```python
from build123d import *

# Parameters (mm, degrees)
BOSS_EXTRUDE1_DEPTH                            = 3
CSK_FOR_M4_FLAT_HEAD_MACHINE_SCREW7_AT_2_COUNT = 2
CSK_FOR_M4_FLAT_HEAD_MACHINE_SCREW7_AT_2_PITCH = 14.1
CSK_FOR_M4_FLAT_HEAD_MACHINE_SCREW7_AT_3_COUNT = 2
CSK_FOR_M4_FLAT_HEAD_MACHINE_SCREW7_AT_3_PITCH = 14.1


with BuildPart() as part:
    # Sketch2 → Boss-Extrude1 (new body)
    with BuildSketch(Plane(origin=(0, 0, 0), x_dir=(1, 0, 0), z_dir=(0, 1, 0))):
        with BuildLine():
            Line((14, -6), (-14, -6))
            ThreePointArc((-14, -6), (-20, 0), (-14, 6))
            Line((-14, 6), (14, 6))
            ThreePointArc((14, 6), (20, 0), (14, -6))
        make_face()
    extrude(amount=-BOSS_EXTRUDE1_DEPTH)

    # Sketch22 → CSK for M4 Flat Head Machine Screw7 (revolve, cut)
    with BuildSketch(Plane(origin=(0, 0, 0), x_dir=(0, 0, 1), z_dir=(1, 0, 0))):
        Polygon((0, 0), (0, 3), (2.25, 3), (2.25, 2.45), (4.7, 0), align=None)
    csk_for_m4_flat_head_machine_screw7 = revolve(axis=Axis((0, 6.35, 0), (0, -1, 0)), mode=Mode.SUBTRACT)

    # CSK for M4 Flat Head Machine Screw7 at 2: CSK for M4 Flat Head Machine Screw7 ×2
    with Locations(*[(-i * CSK_FOR_M4_FLAT_HEAD_MACHINE_SCREW7_AT_2_PITCH, 0, 0) for i in range(1, CSK_FOR_M4_FLAT_HEAD_MACHINE_SCREW7_AT_2_COUNT)]):
        add(csk_for_m4_flat_head_machine_screw7, mode=Mode.SUBTRACT)

    # CSK for M4 Flat Head Machine Screw7 at 3: CSK for M4 Flat Head Machine Screw7 ×2
    with Locations(*[(i * CSK_FOR_M4_FLAT_HEAD_MACHINE_SCREW7_AT_3_PITCH, 0, 0) for i in range(1, CSK_FOR_M4_FLAT_HEAD_MACHINE_SCREW7_AT_3_COUNT)]):
        add(csk_for_m4_flat_head_machine_screw7, mode=Mode.SUBTRACT)


solid = part.part
```
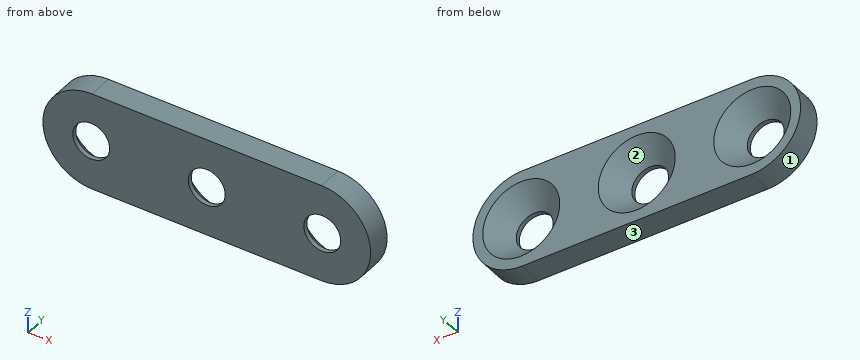
Read the model definition and answer for the solid it produces. Units are mm, in the model's axes. Face numbers are marked on the shaded views. Give positions to 0.01 mm unless a question says otherwise; leave off trailing zeros. Write each loop counter-clockwise with the first axis right and the second up, starting at its lowest first coordinate (ties: lowest second). Pieces come first, ordered by that corner, then holes. Notation, with made-up numbers: (-30, -12.75) - (5, -12.75) arc R20 cw to (5, 13.25) - close; hole circle Ø4 at (72.5, 5). An arc over 180 degrees is marked (long way). Write item = value, one per line. Start each with the question number.
Item 1: Find the intervals of material crossed by probe 1 along X at (y, z) = (-2.7, 0); probe 2 along Z at (x, y) = (14.1, -2.7); probe 3 along X at (y, z) = (-1.7, 1), in increasing order. Write a range as [from, to].
Item 2: Find section A-A (z = 0). Give the vertices of the cut face in (x, y), then the cut area to 3 significant figures.
Item 3: Find section C-C (x = 0). Give the vertices of the cut face in (y, z).
Item 4: Find section B-B (y = -0.6). Give the vertices of the cut face in (x, z).
Item 5: Find section D-D (z = -5.25). Give the vertices of the cut face in (x, y), then the cut area to 3 significant figures.
Item 6: The mould has two halves that part along Z. Classify the marked faces 1, 2 and 3: +Z half, -Z half, draft (parallel to the pull), parting line (faces both ways), or undercut.
Response:
q1.probe_1 = [-20, -16.35], [-11.85, -2.25], [2.25, 11.85], [16.35, 20]
q1.probe_2 = [-6, -2.25], [2.25, 6]
q1.probe_3 = [-19.92, -16.93], [-11.27, -2.83], [2.83, 11.27], [16.93, 19.92]
q2.outline = (-20, -3) - (-16.35, -3) - (-16.35, -2.45) - (-18.8, 0) - (-20, 0) - close; (-11.85, -3) - (-2.25, -3) - (-2.25, -2.45) - (-4.7, 0) - (-9.4, 0) - (-11.85, -2.45) - close; (2.25, -3) - (11.85, -3) - (11.85, -2.45) - (9.4, 0) - (4.7, 0) - (2.25, -2.45) - close; (16.35, -3) - (20, -3) - (20, 0) - (18.8, 0) - (16.35, -2.45) - close
q2.area = 61.5 mm²
q3.outline = (-3, -6) - (0, -6) - (0, -4.7) - (-2.45, -2.25) - (-3, -2.25) - close; (-3, 2.25) - (-2.45, 2.25) - (0, 4.7) - (0, 6) - (-3, 6) - close
q4.outline = (-14, -6) - (14, -6) arc R6 ccw to (14, 6) - (-14, 6) arc R6 ccw to start; hole circle Ø8.2 at (-14.1, 0); hole circle Ø8.2 at (0, 0); hole circle Ø8.2 at (14.1, 0)
q5.outline = (-16.9, -3) - (16.9, -3) - (16.9, 0) - (-16.9, 0) - close
q5.area = 101 mm²
q6.face_1 = parting line
q6.face_2 = undercut
q6.face_3 = -Z half
